The listing builds one solid part. Answer for the finished solid, in the listing's coordinates (mm). Round coordinates to 2 decimals unless told otherwise and drop trailing zeros. Loops run counter-clockwise (first coordinate to the right, second up) from the corner with the lowest first, then second, coordinate; pieces in that order, holes last. Notation, with made-up numbers: M 31.25,-32 L 54.25,-32 A6 ccw 54.25,-28 Z; hole C 0.5,63 d8. An arc over 180 degrees is marked long. Put each result on its own line as item: value. Start each with the question number.
(1) Section B-B, the plane z = 14 is taken. Determine the outline of the cut face in (x, y).
(2) Section A-A, the plane x = 0 is taken. Determine the outline of the cut face in (y, z) (3 decimals).
(3) Flat-ended cylindrical pins translate along their axes: P1, Ø10, axis at x = -9, z = 24, coming from the +Y side; P2, Ø1, axis at y = -8, z = 0.5, coming from the +X side; P3, Ø2, axis at y = -2, z = 40.5, coming from the -X side; P4, Ø5, axis at x = -10, y = -7, coming from the -Z side. Find the tip coordinate at first contact, or state that the pin passes through.
(4) Straight lines are drawn through the part: line 1 (Z direction, x = 0, y = -7.75); line 2 (X direction, y = -7.75, z = -51); line 3 (Z direction, x = 0, y = -11.75). For each, find the intervals that lie inside material, in ascending order.
```python
from build123d import *

# Parameters (mm, degrees)
F1_R      = 16
F2_DEPTH  = 71.1
F3_DEPTH  = 57.1
F3_FACE_R = 16
F5_R      = 12.85
F8_R      = 11.375
F6_FACE_R = 12.85
F10_D     = 12
F10_DEPTH = 16.0010001
F12_D     = 12


with BuildPart() as f2:
    # F1 (on Top) → F2 (new body)
    with BuildSketch(Plane.XY):
        Circle(F1_R)
    extrude(amount=F2_DEPTH)

    # F3 (add): a face of the model
    f3_faces = [f2.faces().sort_by_distance(p)[0] for p in [
        (0, 0, 0),
    ]]
    extrude(f3_faces, amount=F3_DEPTH)

    # F3_face (on face) → F6 section 0
    with BuildSketch(Plane(origin=(0, 0, -57.1), x_dir=(1, 0, 0), z_dir=(0, 0, -1))):
        Circle(F3_FACE_R)
    # F5 (on offset) → F6 section 1
    with BuildSketch(Plane(origin=(0, 0, -69.6), x_dir=(1, 0, 0), z_dir=(0, 0, -1))):
        Circle(F5_R)
    loft()

    # F8 (on offset) → F9 section 0
    with BuildSketch(Plane(origin=(0, 0, -71.35), x_dir=(1, 0, 0), z_dir=(0, 0, -1))):
        Circle(F8_R)
    # F6_face (on face) → F9 section 1
    with BuildSketch(Plane(origin=(0, 0, -69.6), x_dir=(1, 0, 0), z_dir=(0, 0, -1))):
        Circle(F6_FACE_R)
    loft()

    # F10 (through all, one way)
    with BuildSketch(Plane.XZ):
        with Locations((0, -51)):
            Circle(F10_D / 2)
    extrude(amount=-F10_DEPTH, mode=Mode.SUBTRACT)

    # F12 (through all)
    with Locations(Plane(origin=(0, 0, 0), x_dir=(1, 0, 0), z_dir=(0, 1, 0))):
        with Locations((0, 51)):
            Hole(F12_D / 2)


solid = f2.part
```
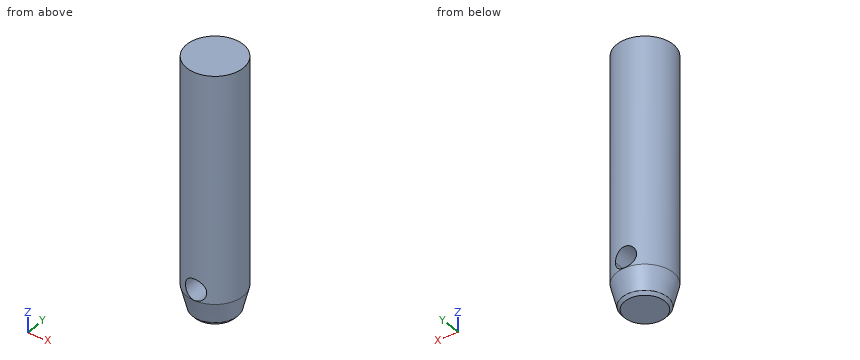
Recorded:
1. outline: C 0,0 d32
2. outline: M -16,-57.1 L -12.85,-69.6 L -11.375,-71.35 L 11.375,-71.35 L 12.85,-69.6 L 16,-57.1 L 16,-57 L -16,-57 Z; M -16,-45 L 16,-45 L 16,71.1 L -16,71.1 Z
3. P1: stops at y = 15.49
3. P2: stops at x = 14.13
3. P3: stops at x = -15.97
3. P4: stops at z = -71.35
4. line 1: z = -71.35 to -57, -45 to 71.1
4. line 2: x = -14 to -6, 6 to 14
4. line 3: z = -70.91 to -57, -45 to 71.1
